Geometry check sheet. Reference: the model listing, model coordinates, mm. A direction names the side the tool comes from. Coordinates: 2 decimals unless noted, no trailing zeros. Write each loop counter-clockwise with the first axis right and the second up, starting at its lowest first coordinate (ties: lowest second). Pieces come first, ordered by that corner, then holes. Notation, with made-up numbers: M 80,53 L 84,53 A21 ccw 84,78 Z; hole C 30.25,3 d9. An arc over 180 degrees is marked long. Put each result on its own line as item: value. Start each with the question number.
1) Gauge pin test, flat ends, axial feed: pin 1 (1.5 mm diameter, centred on y = 2, z = 2, fed in from -X); pin 2 (3.5 mm diameter, centred on x = 29.89, y = 11, fed in from -Z); pin 3 (1.5 mm diameter, centred on y = -2.5, z = 1, fed in from +X); pin 4 (5.5 mm diameter, centred on x = 21, y = 5.83, fed in from +Z). Record the tip position at first contact, or that the pin passes through.
2) Cross-section at C-C on z = 2.5. Record the cut outline in (x, y).
3) Cross-section at D-D on x = -31. Record the cut outline in (y, z), plus the area to 3 significant figures.
4) Set-up check for faces 4 (the flat face through (-26, 0, 1)), 5 (the cylindrical face through (19.3, 5.9, 0.6)), 6 (the flat face through (-26, 22, 1)): record each of +Z, -Z, +X, -X, +Y, -Y from which the full face is reachable in a straight line by a thin tool's end or side.
5) Scan lines: line 1 along X through (y, z) = (11, 2.15); line 2 along Y through (x, z) = (21, 0.55); line 3 along X through (y, z) = (15, 0.8). Record each from-to range of solid material in increasing order.
6) Cross-section at B-B on y = 11. Count the separate pieces of the cut face and the enclosed holes in it, plus the area to 3 significant figures.
7) Mould release check, pull along Y, two halves, no side actions. Record for faces 1 (the cylindrical face through (22.57, 15.35, 0.61)), 2 (the flat face through (-31, 18, 1)), 3 (the flat face through (-4, 11, 3)): released by +Y, released by -Y, zero draft, split by the parting line, or undercut.
8) Cross-section at A-A on x = 6. Record the cut outline in (y, z).
from build123d import *

# Parameters (mm, degrees)
PAD_DEPTH        = 3
SKETCH001_R      = 1.7
POCKET_DEPTH     = 3
SKETCH002_W      = 13
SKETCH002_H      = 3
PAD001_DEPTH     = 10
PAD002_DEPTH     = 10
SKETCH011_R      = 2.3
POCKET003_DEPTH  = 3
POCKET004_DEPTH  = 4
HOLE_D           = 1.75
HOLE_DEPTH       = 14
HOLE_CSINK_D     = 7
HOLE_CSINK_ANGLE = 90


with BuildPart() as part:
    # Sketch → Pad (new body)
    with BuildSketch(Plane.XY):
        Polygon((-26, 26.4999999928), (27.5, 26.4999999928), (27.49902347, -5.4999999923), (-26, -5.5000000072), align=None)
    extrude(amount=PAD_DEPTH)

    # Sketch001 (on Face6 of Pad) → Pocket (cut)
    with BuildSketch(Plane.XY.offset(3)):
        with Locations((6, 16)):
            Circle(SKETCH001_R)
        with Locations((21, 16)):
            Circle(SKETCH001_R)
        with Locations((6, 5.8643429572)):
            Circle(SKETCH001_R)
        with Locations((20.9999664256, 5.8326060428)):
            Circle(SKETCH001_R)
    extrude(amount=-POCKET_DEPTH, mode=Mode.SUBTRACT)

    # Sketch002 (on Face2 of Pocket) → Pad001 (join)
    with BuildSketch(Plane(origin=(-26, 0, 0), x_dir=(0, -1, 0), z_dir=(-1, 0, 0))):
        with Locations((-11.5, 1.5)):
            Rectangle(SKETCH002_W, SKETCH002_H)
    extrude(amount=PAD001_DEPTH)

    # Sketch003 (on Face3 of Pad001) → Pad002 (join)
    with BuildSketch(Plane(origin=(27.4991912855, -0.0008391808, 0), x_dir=(3.05166e-05, 0.9999999995, 0), z_dir=(0.9999999995, -3.05166e-05, 0))):
        Polygon((4.9999999997, -5.34717e-05), (18, 0.0098544685), (18, 3.0102239098), (4.9999999997, 3.0003159696), align=None)
    extrude(amount=PAD002_DEPTH)

    # Sketch011 (on Face10 of Pad002) → Pocket003 (cut)
    with BuildSketch(Plane(origin=(0, 0, 0), x_dir=(1, 0, 0), z_dir=(0, 0, -1))):
        with Locations((-31.3064256507, -11)):
            Circle(SKETCH011_R)
        with Locations((29.8905204819, -11)):
            Circle(SKETCH011_R)
    extrude(amount=-POCKET003_DEPTH, mode=Mode.SUBTRACT)

    # Sketch011 (on Face10 of Pad002) → Pocket004 (cut)
    with BuildSketch(Plane(origin=(0, 0, 0), x_dir=(1, 0, 0), z_dir=(0, 0, -1))):
        with Locations((-31.3064256507, -11)):
            Circle(SKETCH011_R)
        with Locations((29.8905204819, -11)):
            Circle(SKETCH011_R)
    extrude(amount=-POCKET004_DEPTH, mode=Mode.SUBTRACT)

    # Hole
    with Locations(Plane.XY.offset(3)):
        with Locations((6, 16), (21, 16), (6, 5.8643429572), (20.9999664256, 5.8326060428)):
            CounterSinkHole(HOLE_D / 2, HOLE_CSINK_D / 2, depth=HOLE_DEPTH, counter_sink_angle=HOLE_CSINK_ANGLE)


solid = part.part
Answer key:
1. pin 1: stops at x = -26
1. pin 2: passes through
1. pin 3: stops at x = 27.5
1. pin 4: stops at z = 2.25
2. outline: M -36,5 L -26,5 L -26,-5.5 L 27.5,-5.5 L 27.5,5 L 37.5,5 L 37.5,18 L 27.5,18 L 27.5,26.5 L -26,26.5 L -26,18 L -36,18 Z; hole C -31.31,11 d4.6; hole C 6,5.86 d6; hole C 6,16 d6; hole C 21,5.83 d6; hole C 21,16 d6; hole C 29.89,11 d4.6
3. outline: M 5,0 L 8.72,0 L 8.72,3 L 5,3 Z; M 13.28,0 L 18,0 L 18,3 L 13.28,3 Z
3. area: 25.3 mm²
4. face 4: +Z, -Z, -X, -Y
4. face 5: +Z, -Z
4. face 6: +Z, -Z, -X, +Y
5. line 1: x = -36 to -33.61, -29.01 to 27.59, 32.19 to 37.5
5. line 2: y = -5.5 to 4.13, 7.53 to 14.3, 17.7 to 26.5
5. line 3: x = -36 to 4.63, 7.37 to 19.63, 22.37 to 37.5
6. separate pieces: 3
6. enclosed holes: 0
6. area: 193 mm²
7. face 1: undercut
7. face 2: released by +Y
7. face 3: zero draft
8. outline: M -5.5,0 L 4.16,0 L 4.16,1.2 L 2.36,3 L -5.5,3 Z; M 7.56,0 L 14.3,0 L 14.3,1.2 L 12.5,3 L 9.36,3 L 7.56,1.2 Z; M 17.7,0 L 26.5,0 L 26.5,3 L 19.5,3 L 17.7,1.2 Z
